Could you check a few things on this model? Use its own coordinates, in mm. A direction names the side the tool comes from. Round coordinates to 2 decimals unless told otherwise and drop trailing zeros. Loops run counter-clockwise (first coordinate to the right, second up) from the corner with the lowest first, then second, coordinate; pieces in that order, holes last. Notation, with made-up numbers: M 43.5,-21.75 L 62.5,-21.75 A18 ccw 62.5,-8.75 Z; hole C -34.5,60.25 d8. An arc over 180 degrees is marked long. Answer in a Markdown table with one row per item.
```python
from build123d import *

# Parameters (mm, degrees)
F0_R     = 43.929469
F1_DEPTH = 203.2
F2_R     = 17.931427
F3_DEPTH = 228.6
F4_R     = 144.998966
F5_DEPTH = 25.4
F6_R     = 33.658576
F7_DEPTH = 12.7


with BuildPart() as f1:
    # F0 (on Top) → F1 (new body)
    with BuildSketch(Plane.XY):
        Circle(F0_R)
    extrude(amount=F1_DEPTH)

    # F2 (on face) → F3 (join)
    with BuildSketch(Plane.XY.offset(203.2)):
        Circle(F2_R)
    extrude(amount=F3_DEPTH)

    # F4 (on Front) → F5 (join, symmetric)
    with BuildSketch(Plane.XZ):
        Circle(F4_R)
    extrude(amount=F5_DEPTH, both=True)

    # F6 (on face) → F7 (join, symmetric)
    with BuildSketch(Plane.XZ.offset(25.4)):
        with Locations((-76.069236, 54.405343)):
            Circle(F6_R)
    extrude(amount=F7_DEPTH, both=True)


solid = f1.part
```
1) I want a section at B-B, the plane y = 5.5. Please give me the cut outline in (x, z).
Computed:
| item | result |
|---|---|
| outline | M -43.58,138.29 A145 ccw long 43.58,138.29 L 43.58,203.2 L 17.07,203.2 L 17.07,431.8 L -17.07,431.8 L -17.07,203.2 L -43.58,203.2 Z |
2) I need wall thicknesses on line 1 (X direction, y = 1, z = 293.5); line 2 (Y direction, x = 45, z = 38); line 3 (X direction, y = 1, z = 201). Which ranges of each line are inside material? Lowest first, please.
Computed:
| item | result |
|---|---|
| line 1 | x = -17.9 to 17.9 |
| line 2 | y = -25.4 to 25.4 |
| line 3 | x = -43.92 to 43.92 |
3) If we mould it in two halves opening along X, with no side actions, what happens to faces 4 (the face through (-1, -19, 203.2)), 5 (the face through (-102.78, -31.839, 33.925)), 6 (the face through (-3.887, -17.505, 315.9))? For each: released by +X, released by -X, zero draft, split by the parting line, or undercut.
Computed:
| item | result |
|---|---|
| face 4 | zero draft |
| face 5 | undercut |
| face 6 | split by the parting line |
4) Which directions (+Z, -Z, +X, -X, +Y, -Y) give clear straight access to the entire face, cutting with the end or side of a thin tool? Please do faces 1 (the face through (-1, 33, 0)), 2 (the face through (-77, -38.1, 55)), 3 (the face through (-32.38, 29.69, 100.18)).
Computed:
| item | result |
|---|---|
| face 1 | -Z, +X, -X, +Y |
| face 2 | +Z, -Z, -X, -Y |
| face 3 | +Z |
5) I want a section at A-A, the plane x = -63.5. Please give me the cut outline in (y, z).
Computed:
| item | result |
|---|---|
| outline | M -38.1,23.18 L -25.4,23.18 L -25.4,-130.36 L 25.4,-130.36 L 25.4,130.36 L -25.4,130.36 L -25.4,85.63 L -38.1,85.63 Z |
6) Will these pins go through, and if not, where does the flat tip stop? P1, Ø1, axis at x = 63, y = 9, coming from the +Z side; P2, Ø20, axis at x = -86, z = 43, coming from the -Y side; P3, Ø3, axis at y = 10.5, z = 356.5, coming from the -X side.
Computed:
| item | result |
|---|---|
| P1 | stops at z = 130.84 |
| P2 | stops at y = -38.1 |
| P3 | stops at x = -15.51 |
7) I want a section at D-D, the plane x = 0. Please give me the cut outline in (y, z), plus the area to 3 significant figures.
Computed:
| item | result |
|---|---|
| outline | M -43.93,0 L -25.4,0 L -25.4,-145 L 25.4,-145 L 25.4,0 L 43.93,0 L 43.93,203.2 L 17.93,203.2 L 17.93,431.8 L -17.93,431.8 L -17.93,203.2 L -43.93,203.2 Z |
| area | 33,400 mm² |
8) I want a section at C-C, the plane z = 280. Please give me the cut outline in (x, y), plus the area to 3 significant figures.
Computed:
| item | result |
|---|---|
| outline | C 0,0 d35.86 |
| area | 1,010 mm² |
